Here's how the part is built. I have some questions about the finished solid (model axes, mm). A direction names the side the tool comes from. Round coordinates to 2 decimals unless told otherwise and drop trailing zeros. Order: outer loops, then holes, each group sorted by start corner. A loop starts at its lowest first (then second) coordinate and runs counter-clockwise, first axis right, second up. Notation, with made-up numbers: (86.5, 51.5) -> (124.5, 51.5) arc R25 ccw to (124.5, 85.5) -> close; hole circle Ø9 at (27, -2). An arc over 180 degrees is marked (long way). One line per item, written item: value.
```python
from build123d import *

# Parameters (mm, degrees)
SKETCH1_W                       = 20
SKETCH1_H                       = 25
SKETCH1_R                       = 5.1
BOSS_EXTRUDE1_DEPTH             = 6.35
TAP_DRILL_FOR_M3X0_5_TAP1_D     = 2.5
TAP_DRILL_FOR_M3X0_5_TAP3_D     = 2.5
TAP_DRILL_FOR_M3X0_5_TAP3_DEPTH = 6
TAP_DRILL_FOR_M3X0_5_TAP3_TIP   = 0.751075774


with BuildPart() as part:
    # Sketch1 → Boss-Extrude1 (new body)
    with BuildSketch(Plane(origin=(0, 0, 0), x_dir=(1, 0, 0), z_dir=(0, 1, 0))):
        Rectangle(SKETCH1_W, SKETCH1_H)
        with Locations(Location((0, 1.5261946, 0), (0, 0, 270))):
            Circle(SKETCH1_R, mode=Mode.SUBTRACT)
    extrude(amount=BOSS_EXTRUDE1_DEPTH)

    # Tap Drill for M3x0.5 Tap1 (through all)
    with Locations(Plane(origin=(0, 6.35, 0), x_dir=(1, 0, 0), z_dir=(0, 1, 0))):
        with Locations((-8, 1.5261946), (0, 9.5261946), (8, 1.5261946), (0, -6.4738054)):
            Hole(TAP_DRILL_FOR_M3X0_5_TAP1_D / 2)

    # Tap Drill for M3x0.5 Tap3
    with Locations(Plane(origin=(0, 0, -12.5), x_dir=(-1, 0, 0), z_dir=(0, 0, -1))):
        with Locations((-7, 3.175), (7, 3.175)):
            Hole(TAP_DRILL_FOR_M3X0_5_TAP3_D / 2, depth=TAP_DRILL_FOR_M3X0_5_TAP3_DEPTH)
            with Locations((0, 0, -(TAP_DRILL_FOR_M3X0_5_TAP3_DEPTH + TAP_DRILL_FOR_M3X0_5_TAP3_TIP / 2))):  # 118° drill point
                Cone(0, TAP_DRILL_FOR_M3X0_5_TAP3_D / 2, TAP_DRILL_FOR_M3X0_5_TAP3_TIP, mode=Mode.SUBTRACT)


solid = part.part
```
Q1. I need wall thicknesses on line 1 along Y through (x, z) = (-7, -8.8) (3 decimals); line 2 along Z through (x, y) = (8, 2); line 3 along X through (y, z) = (4, 7). Which ranges of each line are inside material? Lowest first, please.
Answers:
line 1: 0 to 1.925, 4.425 to 6.35
line 2: -12.5 to -2.78, -0.28 to 12.5
line 3: -10 to -1.13, 1.13 to 10
Q2. I want a section at C-C on x = -4.5. Write out the boundary of the cut face in (y, z).
Answers:
outline: (0, -12.5) -> (6.35, -12.5) -> (6.35, -3.93) -> (0, -3.93) -> close; (0, 0.87) -> (6.35, 0.87) -> (6.35, 12.5) -> (0, 12.5) -> close
Q3. I want a section at D-D on z = 6. Write out the boundary of the cut face in (x, y), then the cut area to 3 significant figures.
Answers:
outline: (-10, 0) -> (-1.16, 0) -> (-1.16, 6.35) -> (-10, 6.35) -> close; (1.16, 0) -> (10, 0) -> (10, 6.35) -> (1.16, 6.35) -> close
area: 112 mm2
Q4. Which directions (+Z, -Z, +X, -X, +Y, -Y) give clear straight access to the entire face, cutting with the end or side of a thin tool? Please do faces 5 (the face through (-7.92, 4.02, -9.46)), 6 (the face through (10, 3, 0)).
Answers:
face 5: -Z
face 6: +Z, -Z, +X, +Y, -Y
Q5. I want a section at B-B on y = 0.75. Write out the boundary of the cut face in (x, z), then the cut area to 3 significant figures.
Answers:
outline: (-10, -12.5) -> (10, -12.5) -> (10, 12.5) -> (-10, 12.5) -> close; hole circle Ø2.5 at (-8, -1.53); hole circle Ø10.2 at (0, -1.53); hole circle Ø2.5 at (0, -9.53); hole circle Ø2.5 at (0, 6.47); hole circle Ø2.5 at (8, -1.53)
area: 399 mm2
Q6. I want a section at A-A on x = 0. Write out the boundary of the cut face in (y, z), then the cut area to 3 significant figures.
Answers:
outline: (0, -12.5) -> (6.35, -12.5) -> (6.35, -10.78) -> (0, -10.78) -> close; (0, -8.28) -> (6.35, -8.28) -> (6.35, -6.63) -> (0, -6.63) -> close; (0, 3.57) -> (6.35, 3.57) -> (6.35, 5.22) -> (0, 5.22) -> close; (0, 7.72) -> (6.35, 7.72) -> (6.35, 12.5) -> (0, 12.5) -> close
area: 62.2 mm2
Q7. If we mould it in two halves opening along Z, with no side actions, what happens to faces 1 (the face through (6.08, 4.02, -9.46)), 2 (the face through (0, 3, -12.5)), 3 (the face through (1.53, 3.13, 3.34)), 4 (the face through (9.25, 3.13, -1.58))? For each: pulls with the +Z half, pulls with the -Z half, needs draft (parallel to the pull), parting line crosses it, or undercut.
Answers:
face 1: needs draft
face 2: pulls with the -Z half
face 3: undercut
face 4: undercut
Q8. For P1, Ø2, axis at x = -7, y = 3.175, coming from the -Z side, with a flat end and sliding along its axis, tell me the tip position at first contact or that it passes through.
Answers:
P1: z = -6.35
